Work out the finished part from the listing and answer in its coordinate system (mm). Face numbers are marked on the shaded views. A direction names the side the tool comes from. Round coordinates to 2 decimals unless told otherwise and drop trailing zeros. Write each loop counter-clockwise with the first axis right and the second up, starting at its lowest first coordinate (ties: lowest second). Pieces come first, ordered by that corner, then holes. Notation, with made-up numbers: M 30,54 L 43,54 A22 ccw 43,84 Z; hole C 42.5,22 d8. An arc over 180 degrees is marked long. One line per item, written item: value. Start each with the question number.
Q1. Find section A-A (z = 4.5). Write down the section's boundary in (x, y).
Q2. A tool of negligible diameter and unlimited length cuts with its end or side. For the marked faces 5, 6, 7, 8 and 9, from which of +Z, -Z, +X, -X, +Y, -Y can it reach the whole face along a straight path? Write none if from no direction.
Q3. The mould has two halves that part along Y. Classify the marked faces 1, 2, 3 and 4: released by +Y, released by -Y, zero draft, split by the parting line, or undercut.
Q4. Find section B-B (x = 11.75). Write down the section's boundary in (y, z).
Q5. Find section C-C (y = -2.5). Write down the section's boundary in (x, z), and give its area (3 significant figures).
Q6. Consider probe 1 along Y at (x, z) = (20.25, 4); probe 2 along X at (y, z) = (7.25, -7.25); probe 3 along Z at (x, y) = (1.75, 7.75). Determine where each line is inside the solid, lowest interval first.
Q7. Find section D-D (z = -12). Write down the section's boundary in (x, y), and give its area (3 significant figures).
Q8. Given pin 1 Ø4 at (x, z) = (18.5, -7.92) entering from +Y; pin 2 Ø5 at (x, z) = (3.5, -7.92) entering from -Y; pin 3 Ø1.8 at (y, z) = (-6, -8) entering from -X; pin 4 Ø0.6 at (x, y) = (6.5, -4.5) entering from -Z, each flat-ended and moving along its own axis, determine where each tip first touches the part or whether it passes through.
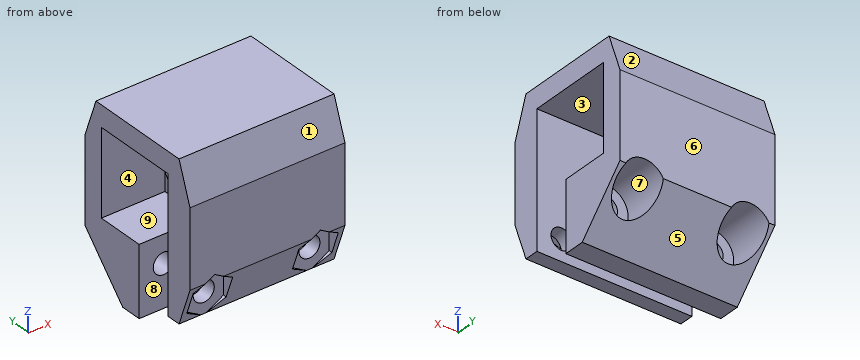
from build123d import *

# Parameters (mm, degrees)
SALIENTE_EXTRUIR1_DEPTH = 22
CROQUIS2_R              = 1.5
CORTAR_EXTRUIR1_DEPTH   = 33.348054431
SALIENTE_EXTRUIR2_START = -9
SALIENTE_EXTRUIR2_DEPTH = 4
CHAFL_N1_SIZE           = 2
CHAFL_N1_SIZE_2         = 5.494954839
CORTAR_EXTRUIR2_DEPTH   = 2
CHAFL_N2_SIZE           = 2
CHAFL_N2_SIZE2          = 5.494954839
CROQUIS5_R              = 3
CORTAR_EXTRUIR3_DEPTH   = 6.9


with BuildPart() as part:
    # Croquis1 → Saliente-Extruir1 (new body)
    with BuildSketch(Plane(origin=(0, 0, 0), x_dir=(0, 0, -1), z_dir=(1, 0, 0))):
        Polygon((0, -3.67871106), (10.9196489, -3.67871106), (10.9196489, -7.67871106), (-11.0803511, -7.67871106), (-11.0803511, 11.52128894), (6.5196489, 11.52128894), (13.9196489, 4.62128894), (13.9196489, 1.62128894), (4.0196489, 1.62128894), (4.0196489, 8.52128894), (-8.0803511, 8.52128894), (-8.0803511, -3.67871106), align=None)
    extrude(amount=SALIENTE_EXTRUIR1_DEPTH)

    # Croquis2 → Cortar-Extruir1 (cut, through all)
    with BuildSketch(Plane.XZ.offset(7.67871106)):
        with Locations(Location((3.5, -7.9196489, 0), (0, 0, 270))):
            Circle(CROQUIS2_R)
        with Locations(Location((18.5, -7.9196489, 0), (0, 0, 270))):
            Circle(CROQUIS2_R)
    extrude(amount=-CORTAR_EXTRUIR1_DEPTH, mode=Mode.SUBTRACT)

    # Croquis3 → Saliente-Extruir2 (add)
    with BuildSketch(Plane(origin=(22, 0, 0), x_dir=(0, 0, -1), z_dir=(1, 0, 0)).offset(SALIENTE_EXTRUIR2_START)):
        with BuildLine():
            Line((-8.0803511, 8.52128894), (-8.0803511, 3.52128894))
            ThreePointArc((-8.0803511, 3.52128894), (-7.378728322, 6.349249529), (-5.436595366, 8.52128894))
            Line((-5.436595366, 8.52128894), (-8.0803511, 8.52128894))
        make_face()
        with BuildLine():
            Line((4.0196489, 8.52128894), (4.0196489, 3.52128894))
            ThreePointArc((4.0196489, 3.52128894), (3.318026122, 6.349249529), (1.375893166, 8.52128894))
            Line((1.375893166, 8.52128894), (4.0196489, 8.52128894))
        make_face()
    extrude(amount=-SALIENTE_EXTRUIR2_DEPTH)

    # Chaflán1
    # the kernel refuses this chamfer: 5.494954839, 2 mm, written as the material it takes off along each edge
    with BuildSketch(Plane(origin=(-14.254982899, -7.67871106, -10.9196489), x_dir=(0, 0.9950833631817486, -0.09904090225205035), z_dir=(1, 0, 0))) as chafl_n1_piece_1:
        Polygon((CHAFL_N1_SIZE * 0.995083363182, CHAFL_N1_SIZE * 0.0990409022521), (-CHAFL_N1_SIZE_2 * 0.0990409022504, CHAFL_N1_SIZE_2 * 0.995083363165), (0, 0), align=None)
    extrude(amount=50.509965797, mode=Mode.SUBTRACT)

    # Croquis4 → Cortar-Extruir2 (cut)
    with BuildSketch(Plane.XZ.offset(7.67871106)):
        Polygon((3.5, -4.686487393), (0.7, -6.303068146), (0.7, -9.536229654), (3.5, -11.152810408), (6.3, -9.536229654), (6.3, -6.303068146), align=None)
        Polygon((18.5, -4.686487393), (15.7, -6.303068146), (15.7, -9.536229654), (18.5, -11.152810408), (21.3, -9.536229654), (21.3, -6.303068146), align=None)
    extrude(amount=-CORTAR_EXTRUIR2_DEPTH, mode=Mode.SUBTRACT)

    # Chaflán2
    chafl_n2_edges = [part.edges().sort_by_distance(p)[0] for p in [
        (11, -7.67871106, 11.0803511),
        (11, 11.52128894, 11.0803511),
    ]]
    chafl_n2_side = [part.faces().sort_by_distance(p)[0] for p in [
        (11, 1.92128894, 11.0803511),
    ]]
    chamfer(chafl_n2_edges, length=CHAFL_N2_SIZE, length2=CHAFL_N2_SIZE2, reference=chafl_n2_side[0])

    # Croquis5 → Cortar-Extruir3 (cut)
    with BuildSketch(Plane(origin=(0, 11.52128894, 0), x_dir=(1, 0, 0), z_dir=(0, 1, 0))):
        with Locations(Location((3.5, 7.9196489, 0), (0, 0, 270))):
            Circle(CROQUIS5_R)
        with Locations(Location((18.5, 7.9196489, 0), (0, 0, 270))):
            Circle(CROQUIS5_R)
    extrude(amount=-CORTAR_EXTRUIR3_DEPTH, mode=Mode.SUBTRACT)


solid = part.part
The answers:
1. outline: M 0,-7.68 L 22,-7.68 L 22,-3.68 L 0,-3.68 Z; M 0,8.52 L 22,8.52 L 22,11.52 L 0,11.52 Z
2. face 5: -Z, +X, -X, +Y
2. face 6: +Z, -Z, +X, -X, +Y
2. face 7: +Y
2. face 8: -Z, +X, -X
2. face 9: none
3. face 1: released by -Y
3. face 2: released by +Y
3. face 3: undercut
3. face 4: undercut
4. outline: M -7.68,-5.42 L -5.68,-10.92 L -3.68,-10.92 L -3.68,8.08 L 3.52,8.08 A6.05 cw 8.52,5.44 L 8.52,-1.38 A6.05 cw 3.52,-4.02 L 1.62,-4.02 L 1.62,-13.92 L 4.62,-13.92 L 11.52,-6.52 L 11.52,5.59 L 9.52,11.08 L -5.68,11.08 L -7.68,5.59 Z
5. outline: M 0,8.08 L 22,8.08 L 22,11.08 L 0,11.08 Z
5. area: 66.0 mm2
6. probe 1: -7.68 to -3.68, 8.52 to 11.52
6. probe 2: 0 to 0.58, 6.42 to 15.58, 21.42 to 22
6. probe 3: -10.56 to -10.36, -5.48 to -4.02, 8.08 to 11.08
7. outline: M 0,1.62 L 22,1.62 L 22,6.41 L 0,6.41 Z
7. area: 105 mm2
8. pin 1: y = 4.62
8. pin 2: y = -5.68
8. pin 3: x = 0
8. pin 4: z = -10.92
